Source: CAD feature listing. Evaluate the final solid. Frame: model axes, mm. A direction names the side the tool comes from. Coordinates: 2 decimals unless noted, no trailing zeros. Loops run counter-clockwise (first coordinate to the right, second up) from the corner with the lowest first, then second, coordinate; pieces in that order, holes last.
Item 1: Section query B-B, the plane y = -321. Return the cut outline in (x, z).
Item 2: Section query A-A, the plane z = 0. Return the cut outline in (x, y), then the cut area to 3 significant figures.
Item 3: Reachability of faces 1 (the cylindrical face through (15.929, -228.15, 5.016)), 2 (the cylindrical face through (-12.23, -11.37, 7.5)) from +Z, -Z, +X, -X, +Y, -Y: full face, straight path, thin tool, end or side. Return the list, or none.
Item 4: Section query C-C, the plane x = -59.5. Return the cut outline in (y, z).
Item 5: Pin query (flat end, axial travel): pin 1 Ø4 at (y, z) = (-266, -10) entering from -X; pin 2 Ø2 at (y, z) = (-74, -8) entering from -X; pin 3 Ø12 at (y, z) = (-202, -13.5) entering from +X. Return the tip coordinate at first contact, or that it passes through.
Item 6: Line query: probe 1 along Z at (x, y) = (-1, -115); probe 2 along X at (y, z) = (-300, 1.5); probe 3 along Y at (x, z) = (-59.5, 4.5). Output: solid intervals per line, ascending.
Item 7: Pull-direction query (Y, two-part tool) for faces 3 (the cylindrical face through (12.87, -232.69, -5.34)), 4 (the cylindrical face through (-57.6, -513.29, 4.18)), 5 (the cylindrical face through (-57.605, -515.427, -6.396)); classes: +Y half, -Y half, draft (parallel to the pull), parting line (faces both ways), or undercut.
```python
from build123d import *

# Parameters (mm, degrees)
F1_R          = 16.7
F1_R_2        = 13.932
F3_R          = 16.7
F4_DEPTH      = 25
F4_DEPTH_BACK = 25


with BuildPart() as f2:
    # F2: sweep along a path in F0
    with BuildLine(Plane.XY) as f2_path:
        Line((0, 0), (0, -450))
        ThreePointArc((0, -450), (-14.6446609407, -485.3553390593), (-50, -500))
        Line((-50, -500), (-65, -500))
    # F1 (on Front) → F2 (sweep)
    with BuildSketch(Plane.XZ):
        Circle(F1_R)
        Circle(F1_R_2, mode=Mode.SUBTRACT)
    sweep(path=f2_path.line)

    # F3 (on Top) → F4 (cut, two sides)
    with BuildSketch(Plane.XY) as f4_sk:
        Circle(F3_R)
    extrude(amount=-F4_DEPTH, mode=Mode.SUBTRACT)
    extrude(f4_sk.sketch, amount=F4_DEPTH_BACK, mode=Mode.SUBTRACT)


solid = f2.part
```
Verdict:
1. outline: circle Ø33.4 at (0, 0); hole circle Ø27.86 at (0, 0)
2. outline: (-65, -516.7) - (-50, -516.7) arc R66.7 ccw to (16.7, -450) - (16.7, 0) arc R16.7 cw to (13.93, -9.21) - (13.93, -450) arc R63.93 cw to (-50, -513.93) - (-65, -513.93) - close; (-65, -486.07) - (-50, -486.07) arc R36.07 ccw to (-13.93, -450) - (-13.93, -9.21) arc R16.7 cw to (-16.7, 0) - (-16.7, -450) arc R33.3 cw to (-50, -483.3) - (-65, -483.3) - close
2. area: 2,970 mm2
3. face 1: +Y
3. face 2: +Z, -Z, +Y
4. outline: circle Ø33.4 at (-500, 0); hole circle Ø27.86 at (-500, 0)
5. pin 1: stops at x = -14.66
5. pin 2: stops at x = -15.16
5. pin 3: stops at x = 14.92
6. probe 1: z = -16.67 to -13.9, 13.9 to 16.67
6. probe 2: x = -16.63 to -13.85, 13.85 to 16.63
6. probe 3: y = -516.08 to -513.19, -486.81 to -483.92
7. face 3: draft
7. face 4: undercut
7. face 5: parting line
